Can you work these out from the model? Positions are in its coordinate system, mm. A direction names the side the tool comes from. Coordinates: 2 decimals unless noted, no trailing zeros. Order: outer loops, then holes, each group sorted by start corner. A loop starts at its lowest first (then second) coordinate and runs counter-clockwise, first axis right, second up. Notation, with made-up numbers: (15, -6.75) - (32, -6.75) arc R29 cw to (32, 17.25) - close; hole circle Ø11 at (5.25, 50.25). An arc over 180 degrees is marked (long way). Return JSON: item names as keys, results as strings. Group by question number.
1) Imagine slicing it at B-B (z = 23). Write out the boundary of the cut face in (x, y), and give its area (3 significant figures).
2) Imagine slicing it at D-D (z = 71). Write out the boundary of the cut face in (x, y), and give its area (3 significant figures).
3) Imagine slicing it at C-C (x = 19.5). Write out the boundary of the cut face in (y, z), and give its area (3 significant figures).
4) For pin 1 Ø2 at (y, z) = (-365.5, 8.5) entering from +X; pin 2 Ø2 at (x, y) = (46, -220) entering from +Z; pin 3 Ø10 at (x, z) = (34.5, 2.5) entering from -Y, each with a flat end and sliding along its axis, tell me the tip position at first contact or that it passes through.
5) If we mould it in two halves opening along Y, with no side actions, what happens to faces 3 (the face through (41, -304.8, 3)), 4 (the face through (6.35, -232, 47)), 5 (the face through (3.219, -46.233, 13.434))? For each: pulls with the +Y half, pulls with the -Y half, needs draft (parallel to the pull), parting line crosses it, or undercut.
6) Imagine slicing it at A-A (y = -312.5). Write out the boundary of the cut face in (x, z).
7) If I drill on line 1 along X through (y, z) = (-270, 59.5); line 2 along X through (y, z) = (-88, 5), over which ranges is the centre line in solid material (lowest first)?
8) Which directions (+Z, -Z, +X, -X, +Y, -Y) give clear straight access to the entire face, cutting with the end or side of a thin tool? Please do faces 1 (the face through (42, -150, 6.35)), 2 (the face through (3.2, -235.4, 30.8)).
```python
from build123d import *

# Parameters (mm, degrees)
F0_W        = 76.2
F0_H        = 304.8
F1_DEPTH    = 6.35
F2_W        = 457.2
F2_H        = 76.2
F3_DEPTH    = 6.35
F4_R        = 5.08
F5_T1_DEPTH = 304.8
F6_R        = 9.525
F7_DEPTH    = 25.4
F8_R        = 9.525
F9_DEPTH    = 25.4
F10_R       = 9.525
F11_DEPTH   = 25.4
F12_R       = 9.525
F13_DEPTH   = 25.4
F14_R       = 25.4
F15_DEPTH   = 25.4


# Not quite as in the source:
# - a fillet or chamfer that OpenCascade refuses, or shapes differently, is made with other operations: its cross-section is extruded or revolved along the edge and cut away or added


with BuildPart() as f1:
    # F0 (on Top) → F1 (new body)
    with BuildSketch(Plane.XY):
        with Locations((38.1, -152.4)):
            Rectangle(F0_W, F0_H)
    extrude(amount=F1_DEPTH)

    # F2 (on Right) → F3 (join)
    with BuildSketch(Plane.YZ):
        with Locations((-228.6, 38.1)):
            Rectangle(F2_W, F2_H)
    extrude(amount=F3_DEPTH)

    # F4
    f4_edges = [f1.edges().sort_by_distance(p)[0] for p in [
        (0, -228.6, 0),
    ]]
    fillet(f4_edges, radius=F4_R)

    # F5: fillet of radius 2.54 on 1 edges, made by hand

    # F5_s2 → F5_t1 (join)
    with BuildSketch(Plane.XZ):
        with BuildLine():
            add(Edge.make_bspline(
                [(8.89, 6.35), (6.35, 6.35), (6.35, 8.89)],
                knots=[0, 0, 0, 1, 1, 1], degree=2, weights=[1, 1, 1]))
            Line((6.35, 8.89), (6.35, 6.35))
            Line((6.35, 6.35), (8.89, 6.35))
        make_face()
    extrude(amount=F5_T1_DEPTH)

    # F6 (on face) → F7 (cut)
    with BuildSketch(Plane.YZ.offset(6.35)):
        with Locations((-284.6438884735, 37.907961756)):
            Circle(F6_R)
    extrude(amount=-F7_DEPTH, mode=Mode.SUBTRACT)

    # F8 (on face) → F9 (cut)
    with BuildSketch(Plane.YZ.offset(6.35)):
        with Locations((-258.5102617741, 39.1981378198)):
            Circle(F8_R)
    extrude(amount=-F9_DEPTH, mode=Mode.SUBTRACT)

    # F10 (on face) → F11 (cut)
    with BuildSketch(Plane.YZ.offset(6.35)):
        with Locations((-227.8595268726, 36.6169922054)):
            Circle(F10_R)
    extrude(amount=-F11_DEPTH, mode=Mode.SUBTRACT)

    # F12 (on face) → F13 (cut)
    with BuildSketch(Plane.YZ.offset(6.35)):
        with Locations((-196.8858391047, 36.2943448126)):
            Circle(F12_R)
    extrude(amount=-F13_DEPTH, mode=Mode.SUBTRACT)

    # F14 (on face) → F15 (cut)
    with BuildSketch(Plane.YZ.offset(6.35)):
        with Locations((-40.7262966037, 38.2302068174)):
            Circle(F14_R)
    extrude(amount=-F15_DEPTH, mode=Mode.SUBTRACT)


solid = f1.part
```
Calculated:
{
 "1": {"outline": "(0, -457.2) - (6.35, -457.2) - (6.35, -61.05) - (0, -61.05) - close; (0, -20.4) - (6.35, -20.4) - (6.35, 0) - (0, 0) - close", "area": "2,650 mm2"},
 "2": {"outline": "(0, -457.2) - (6.35, -457.2) - (6.35, 0) - (0, 0) - close", "area": "2,900 mm2"},
 "3": {"outline": "(-304.8, 0) - (0, 0) - (0, 6.35) - (-304.8, 6.35) - close", "area": "1,940 mm2"},
 "4": {"pin 1": "x = 6.35", "pin 2": "z = 6.35", "pin 3": "y = -304.8"},
 "5": {"face 3": "pulls with the -Y half", "face 4": "needs draft", "face 5": "undercut"},
 "6": {"outline": "(0, 5.08) arc R5.08 ccw to (5.08, 0) - (6.35, 0) - (6.35, 76.2) - (0, 76.2) - close"},
 "7": {"line 1": "0 to 6.35", "line 2": "0 to 76.2"},
 "8": {"face 1": "+Z, +X, +Y, -Y", "face 2": "+X, -X"}
}
